```python
from build123d import *

# Parameters (mm, degrees)
F0_W     = 3.048
F0_H     = 5.588
F0_R     = 1.4732
F1_DEPTH = 25.4


with BuildPart() as f1:
    # F0 (on Right) → F1 (new body)
    with BuildSketch(Plane.YZ):
        Polygon((-44.894837, -69.046037), (-72.387907, -69.046037), (-72.387907, -145.246037), (-19.555907, -145.246037), (-19.555907, -142.299637), (-15.314107, -142.299637), (-15.314107, -135.647137), (-16.965107, -135.647137), (-16.965107, -132.395937), (-15.314107, -132.395937), (-15.314107, -128.585937), (-12.367707, -128.585937), (-12.367707, -132.395937), (-10.716707, -132.395937), (-10.716707, -135.647137), (-12.367707, -135.647137), (-12.367707, -142.124137), (-8.125907, -142.124137), (-8.125907, -145.070537), (20.322093, -145.070537), (20.322093, -142.316303), (24.563893, -142.316303), (24.563893, -135.839303), (22.912893, -135.839303), (22.912893, -132.588103), (24.563893, -132.588103), (24.563893, -128.778103), (27.510293, -128.778103), (27.510293, -132.588103), (29.161293, -132.588103), (29.161293, -135.839303), (27.510293, -135.839303), (27.510293, -142.316303), (31.752093, -142.316303), (31.752093, -145.495363), (54.612093, -145.495363), (54.612093, -129.683863), (51.644098, -129.683863), (51.647506, -123.079863), (46.049349, -123.079863), (46.049349, -124.730863), (42.798149, -124.730863), (42.798149, -123.079863), (38.988149, -123.079863), (38.988149, -120.133463), (42.798149, -120.133463), (42.798149, -118.482463), (46.049349, -118.482463), (46.049349, -120.133463), (51.694974, -120.133463), (51.694974, -115.053463), (54.641374, -115.053463), (54.641374, -99.483097), (51.665693, -99.483097), (51.665693, -93.642298), (45.188693, -93.642298), (45.188693, -95.296937), (41.937493, -95.296937), (41.937493, -93.645937), (38.127493, -93.645937), (38.127493, -90.699537), (41.937493, -90.699537), (41.937493, -89.048537), (45.188693, -89.048537), (45.188693, -90.699537), (51.665693, -90.699537), (51.665693, -84.857537), (54.612093, -84.857537), (54.612093, -71.992437), (54.612093, -69.046037), (31.752093, -69.046037), (31.752093, -71.992437), (27.478132, -71.992437), (27.478132, -78.469437), (29.129132, -78.469437), (29.129132, -81.720637), (27.478132, -81.720637), (27.478132, -85.530637), (24.531732, -85.530637), (24.531732, -81.720637), (22.782468, -81.720637), (22.782468, -78.469437), (24.433468, -78.469437), (24.433468, -71.992437), (20.322093, -71.992437), (20.322093, -69.046037), (-8.125907, -69.046037), (-8.125907, -71.992437), (-12.494707, -71.992437), (-12.494707, -78.469437), (-10.843707, -78.469437), (-10.843707, -81.720637), (-12.494707, -81.720637), (-12.494707, -85.530637), (-15.441107, -85.530637), (-15.441107, -81.720637), (-17.092107, -81.720637), (-17.092107, -78.469437), (-15.441107, -78.469437), (-15.441107, -71.992437), (-19.555907, -71.992437), (-19.555907, -69.046037), align=None)
        with Locations((-43.431907, -126.958037)):
            Rectangle(F0_W, F0_H, mode=Mode.SUBTRACT)
        with Locations((6.098093, -143.343337)):
            Circle(F0_R, mode=Mode.SUBTRACT)
        with Locations((-43.431907, -87.334037)):
            Rectangle(F0_W, F0_H, mode=Mode.SUBTRACT)
        with Locations((52.914174, -107.268363)):
            Circle(F0_R, mode=Mode.SUBTRACT)
        Polygon((-60.623973, -75.769594), (-62.216802, -77.766938), (-64.771501, -77.766938), (-66.36433, -75.769594), (-65.795856, -73.278946), (-63.494152, -72.170503), (-61.192447, -73.278946), align=None, mode=Mode.SUBTRACT)
        with Locations((6.098093, -70.773237)):
            Circle(F0_R, mode=Mode.SUBTRACT)
    extrude(amount=F1_DEPTH)


with BuildPart() as f1_1:
    # F2: moved
    add(f1.part.moved(Location((0, -1.524, -27.432))))


solid = f1_1.part
```
Work out the finished part from the listing and answer in its coordinate system (mm). A direction names the side the tool comes from. Round coordinates to 2 decimals unless told otherwise and drop trailing zeros. Order: outer loops, then holes, each group sorted by start corner. A loop starts at its lowest first (then second) coordinate and runs counter-clockwise, first axis right, second up.
Q1. A cutting plane is placed at A-A, the plane z = -164.5. Determine the outline of the cut face in (x, y).
Solution:
outline: (0, -73.91) - (25.4, -73.91) - (25.4, -16.84) - (0, -16.84) - close; (0, -13.89) - (25.4, -13.89) - (25.4, 23.04) - (0, 23.04) - close; (0, 25.99) - (25.4, 25.99) - (25.4, 53.09) - (0, 53.09) - close
Q2. A cutting plane is placed at C-C, the plane z = -124. Determine the outline of the cut face in (x, y).
Solution:
outline: (0, -73.91) - (25.4, -73.91) - (25.4, 50.14) - (0, 50.14) - close
Q3. A tool of negligible diameter and unlimited length cuts with its end or side. For faces 5 (the flat face through (13, -16.965, -103)), 6 (the flat face through (13, -12.368, -108)), 7 (the flat face through (13, 23.04, -167)), from which of +Z, -Z, +X, -X, +Y, -Y can it reach the whole face along a straight path? Write none if from no direction.
Solution:
face 5: +Z, +X, -X
face 6: +X, -X
face 7: -Z, +X, -X
Q4. The mould has two halves that part along Z. Classify faces 1 (the flat face through (13, 21.389, -162)), 2 (the flat face through (13, 21, -169.748)), 3 (the flat face through (13, -73.912, -134)), 4 (the flat face through (13, -45, -151.596)): pulls with the +Z half, pulls with the -Z half, needs draft (parallel to the pull), parting line crosses it, or undercut.
Solution:
face 1: undercut
face 2: pulls with the -Z half
face 3: needs draft
face 4: undercut
Q5. Given pin 1 Ø12.5 at (x, z) = (9.5, -104.5) entering from +Y; pin 2 Ø0.8 at (x, y) = (7, -18) entering from -Z; pin 3 Ø0.9 at (x, z) = (18, -119) entering from +Y, each flat-ended and moving along its own axis, determine where each tip first touches the part or whether it passes through.
Solution:
pin 1: stops at y = 53.09
pin 2: stops at z = -169.73
pin 3: stops at y = 36.6
Q6. A cutting plane is placed at D-D, the plane x = 21.5. Count the separate pieces of the cut face and the enclosed holes in it, then the cut area to 3 significant figures.
Solution:
separate pieces: 1
enclosed holes: 6
area: 9,080 mm2
Q7. Find the intervals of material crossed by line 1 along Y through (x, z) = (23.25, -106); line 2 along Y through (x, z) = (5, -163.5); line 3 along Z through (x, y) = (1.75, -45.5), in increasing order.
Solution:
line 1: y = -73.91 to -18.62, -12.37 to 21.26, 27.61 to 53.09
line 2: y = -73.91 to -16.84, -13.89 to 23.04, 25.99 to 53.09
line 3: z = -172.68 to -157.18, -151.6 to -117.56, -111.97 to -96.48
Q8. A cutting plane is placed at B-B, the plane z = -154. Determine the outline of the cut face in (x, y).
Solution:
outline: (0, -73.91) - (25.4, -73.91) - (25.4, -46.48) - (0, -46.48) - close; (0, -43.43) - (25.4, -43.43) - (25.4, 50.12) - (0, 50.12) - close
